Part model, mm, in its own coordinate system. Face numbers are marked on the shaded views. A direction names the side the tool comes from. Round coordinates to 2 decimals unless told otherwise and drop trailing zeros. Loops run counter-clockwise (first coordinate to the right, second up) from the corner with the lowest first, then second, coordinate; pieces in that order, holes last. Notation, with made-up numbers: (43, 61.25) - (63, 61.25) arc R24 cw to (63, 88.25) - close; hole circle Ø11 at (74.25, 46.25). An arc over 180 degrees is marked (long way). Put each result on its own line as item: value.
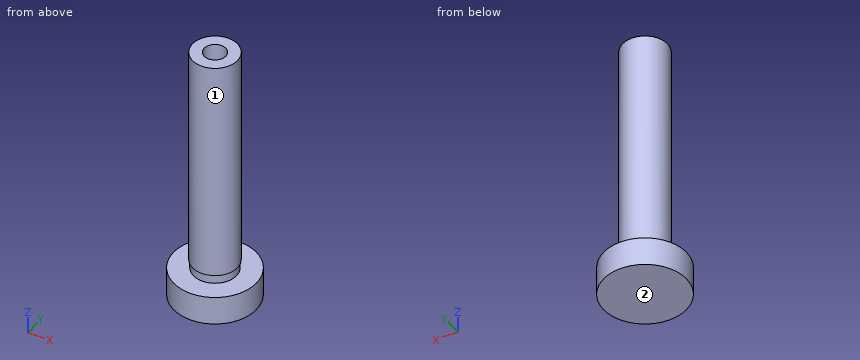
Autodesk Inventor part; units mm, degrees
ref_plane "YZ Plane" through (0, 0, 0) normal (1, 0, 0) x (0, 1, 0)
ref_plane "XZ Plane" through (0, 0, 0) normal (0, 1, 0) x (-1, 0, 0)
ref_plane "XY Plane" through (0, 0, 0) normal (0, 0, 1) x (1, 0, 0)
sketch "Sketch1" plane through (0, 0, 0) normal (0, 0, 1) x (1, 0, 0)
  circle A0 centre (0, 0) radius 23
  dimension "d0" = 46
extrude "Extrusion1" add sketch "Sketch1" along normal blind 16
sketch "Sketch2" plane through (0, 0, 16) normal (0, 0, 1) x (1, 0, 0)
  circle A0 centre (0, 0) radius 12.5
  dimension "d3" = 25
extrude "Extrusion2" add sketch "Sketch2" along normal blind 130
sketch "Sketch3" plane through (0, 0, 146) normal (0, 0, 1) x (1, 0, 0)
  circle A0 centre (0, 0) radius 6
  dimension "d6" = 12
extrude "Extrusion3" cut sketch "Sketch3" against normal blind 25
sketch "Sketch4" plane through (0, 0, 121) normal (0, 0, 1) x (1, 0, 0)
  circle A0 centre (0, 0) radius 12.5
  circle A1 centre (0, 0) radius 7
  dimension "d9" = 14
extrude "Extrusion4" cut sketch "Sketch4" against normal blind 6 contours A1
sketch "Sketch5" plane through (0, 0, 0) normal (0, 1, 0) x (-1, 0, 0)
  line L0 (12.5, 16) -> (12.5, 146)
  line L1 (12.5, 16) -> (12, 16)
  line L2 (12, 16) -> (12, 21)
  line L3 (12, 21) -> (12.5, 21)
  line L4 (12.5, 21) -> (12.5, 16)
  line L5 (23, 16) -> (-23, 16)
  line L6 (0, -4.7692) -> (0, 158.9515) construction
  point P0 (0, 0)
  dimension "d12" = 0.5
  dimension "d13" = 5
  dimension "d14" = 0
revolve "Revolution1" cut sketch "Sketch5" angle 360 about axis through (0, 0, -4.7692) along (0, 0, 1)
properties part number "Pino do Amassador"
1. Tool access for the marked faces 1 and 2: list every direction of +Z, -Z, +X, -X, +Y, -Y with a clear straight run to the whole face (end or side of a thin tool).
A:
face 1: +Z
face 2: -Z, +X, -X, +Y, -Y
2. Pin check, flat tips, straight feed: P1, Ø10, axis at y = -16.5, z = 101.5, coming from the -X side; P2, Ø5, axis at y = -8, z = 84, coming from the +X side (3 decimals); P3, Ø6, axis at y = -11.5, z = 39, coming from the -X side. Stop position of each tip, or through.
A:
P1: stops at x = -4.9
P2: stops at x = 11.225
P3: stops at x = -9.17
3. Band-saw the part on C-C (z = 127). List the corners of the cut face in (x, y).
A:
outline: circle Ø25 at (0, 0); hole circle Ø12 at (0, 0)
4. Band-saw the part on D-D (z = 23). List the corners of the cut face in (x, y).
A:
outline: circle Ø25 at (0, 0)
5. Band-saw the part on A-A (x = 0). List the corners of the cut face in (y, z), plus the area to 3 significant figures.
A:
outline: (-23, 0) - (23, 0) - (23, 16) - (12, 16) - (12, 21) - (12.5, 21) - (12.5, 146) - (6, 146) - (6, 121) - (7, 121) - (7, 115) - (-7, 115) - (-7, 121) - (-6, 121) - (-6, 146) - (-12.5, 146) - (-12.5, 21) - (-12, 21) - (-12, 16) - (-23, 16) - close
area: 3,600 mm²
6. Probe line 1 along Z through (x, y) = (6, -2); line 2 along Y through (x, z) = (0, 137); line 3 along Z through (x, y) = (-15, -2.5). List the from-to ranges inside material, lowest first. Write a range as [from, to].
A:
line 1: z = [0, 115], [121, 146]
line 2: y = [-12.5, -6], [6, 12.5]
line 3: z = [0, 16]
